CAD build for the part. Positions are in the model's coordinates, mm. A direction names the side the tool comes from. Coordinates: 2 decimals unless noted, no trailing zeros. Write each loop counter-clockwise with the first axis right and the second up, starting at its lowest first coordinate (ties: lowest second). Pieces come first, ordered by that corner, then holes. Notation, with made-up numbers: (-37, 48.25) - (-9, 48.25) arc R14 ccw to (-9, 52.25) - close; hole circle Ø6 at (48, 10). An arc over 180 degrees is marked (long way). One line per question, with ' | ' between items. Start each with the question number.
1. Two-plate mould, pull along X, no slides. Class faces 4 (the cylindrical face through (37.746, -3.755, 11.923)), 5 (the cylindrical face through (-28.39, -0.09, 10.47)), 6 (the flat face through (123.945, -9, -9)): +X half, -X half, draft (parallel to the pull), parting line (faces both ways), or undercut.
2. Band-saw the part on A-A, the plane x = -20. Write the cut outline in (y, z), then the cut area to 3 significant figures.
3. Probe line 1 (Y direction, x = -25, z = -11); line 2 (X direction, y = -1, z = -11.5); line 3 (Y direction, x = 9.5, z = 10.5). List the from-to ranges inside material, lowest first.
4. Band-saw the part on B-B, the plane z = 0. Write the cut outline in (x, y), then the cut area to 3 significant figures.
5. Flat gauge pins, fed straight in: P1, Ø5, axis at x = 2.5, y = -4.5, coming from the -Z side; P2, Ø8, axis at x = 41, z = 11.5, coming from the +Y side; P3, Ø1.7, axis at x = -14, z = 10, coming from the -Y side. Where does each tip first touch, or does it go through?
6. Band-saw the part on D-D, the plane x = 14. Write the cut outline in (y, z).
7. Which spindle directions (+Z, -Z, +X, -X, +Y, -Y) get a long thin tool onto all of the face, cutting with end or side? Do faces 1 (the cylindrical face through (11.607, 0.088, 10.472)), 2 (the cylindrical face through (-18.75, 11.09, 5.77)), 3 (the cylindrical face through (11.607, 0.088, -10.533)). Say none if no direction does.
from build123d import *

# Parameters (mm, degrees)
IZIM2_W               = 1.3
IZIM2_H               = 1.828643919
KES_EKSTR_ZYON1_START = 8.5
KES_EKSTR_ZYON1_DEPTH = 10
KES_EKSTR_ZYON2_START = -18.5
KES_EKSTR_ZYON2_DEPTH = 10


with BuildPart() as part:
    # izim1 → D_nd_r1 (revolve)
    with BuildSketch(Plane.XY, mode=Mode.PRIVATE) as d_nd_r1_sk:
        Polygon((0, 0), (-61, 0), (-61, 10.5), (-59, 12.5), (1.944879757, 12.5), (51.944879757, 12.5), (51.944879757, 17), (123.944879757, 17), (123.944879757, 12.5), (183.944879757, 12.5), (183.944879757, 0), (123.944879757, 0), align=None)
    revolve(d_nd_r1_sk.sketch.rotate(Axis((0, 0, 0), (1, 0, 0)), 90), axis=Axis((0, 0, 0), (1, 0, 0)))

    # izim2 → Kes-D_nd_r1 (revolve, cut)
    with BuildSketch(Plane(origin=(0, 0, 0), x_dir=(1, 0, 0), z_dir=(0, 1, 0))):
        with Locations((23.29, -12.864321959)):
            Rectangle(IZIM2_W, IZIM2_H)
    revolve(axis=Axis((0, 0, 0), (1, 0, 0)), mode=Mode.SUBTRACT)

    # izim3 → Kes-Ekstr_zyon1 (cut)
    with BuildSketch(Plane.XY.offset(KES_EKSTR_ZYON1_START)):
        with BuildLine():
            Line((-24.391699554, 4), (7.608300446, 4))
            ThreePointArc((7.608300446, 4), (11.608300446, 0), (7.608300446, -4))
            Line((7.608300446, -4), (-24.391699554, -4))
            ThreePointArc((-24.391699554, -4), (-28.391699554, 0), (-24.391699554, 4))
        make_face()
    extrude(amount=KES_EKSTR_ZYON1_DEPTH, mode=Mode.SUBTRACT)

    # izim3_2 → Kes-Ekstr_zyon2 (cut)
    with BuildSketch(Plane.XY.offset(KES_EKSTR_ZYON2_START)):
        with BuildLine():
            Line((-24.391699554, 4), (7.608300446, 4))
            ThreePointArc((7.608300446, 4), (11.608300446, 0), (7.608300446, -4))
            Line((7.608300446, -4), (-24.391699554, -4))
            ThreePointArc((-24.391699554, -4), (-28.391699554, 0), (-24.391699554, 4))
        make_face()
    extrude(amount=KES_EKSTR_ZYON2_DEPTH, mode=Mode.SUBTRACT)


solid = part.part
Filled in:
1) face 4: draft | face 5: undercut | face 6: +X half
2) outline: (-4, -11.84) - (-4, -8.5) - (4, -8.5) - (4, -11.84) arc R12.5 ccw to (4, 11.84) - (4, 8.5) - (-4, 8.5) - (-4, 11.84) arc R12.5 ccw to start | area: 430 mm²
3) line 1: y = -5.94 to -3.95, 3.95 to 5.94 | line 2: x = -59.96 to -28.26, 11.48 to 183.94 | line 3: y = -6.78 to -3.52, 3.52 to 6.78
4) outline: (-61, -10.5) - (-59, -12.5) - (22.64, -12.5) - (22.64, -11.95) - (23.94, -11.95) - (23.94, -12.5) - (51.94, -12.5) - (51.94, -17) - (123.94, -17) - (123.94, -12.5) - (183.94, -12.5) - (183.94, 12.5) - (123.94, 12.5) - (123.94, 17) - (51.94, 17) - (51.94, 12.5) - (23.94, 12.5) - (23.94, 11.95) - (22.64, 11.95) - (22.64, 12.5) - (-59, 12.5) - (-61, 10.5) - close | area: 6,770 mm²
5) P1: stops at z = -11.84 | P2: stops at y = 10 | P3: stops at y = -8.52
6) outline: circle Ø25 at (0, 0)
7) face 1: +Z | face 2: -X | face 3: -Z
